The figure shows three views and two pictorial views of one solid part (mm, origin at its lowest corner). Answer the questions. Coordinates: 2 decimals unless noted, no trailing zeros. Write each loop counter-clockwise with the first axis right and the second up, starting at its lowest first coordinate (ties: lowest second). Pieces come first, ordered by that corner, then holes.
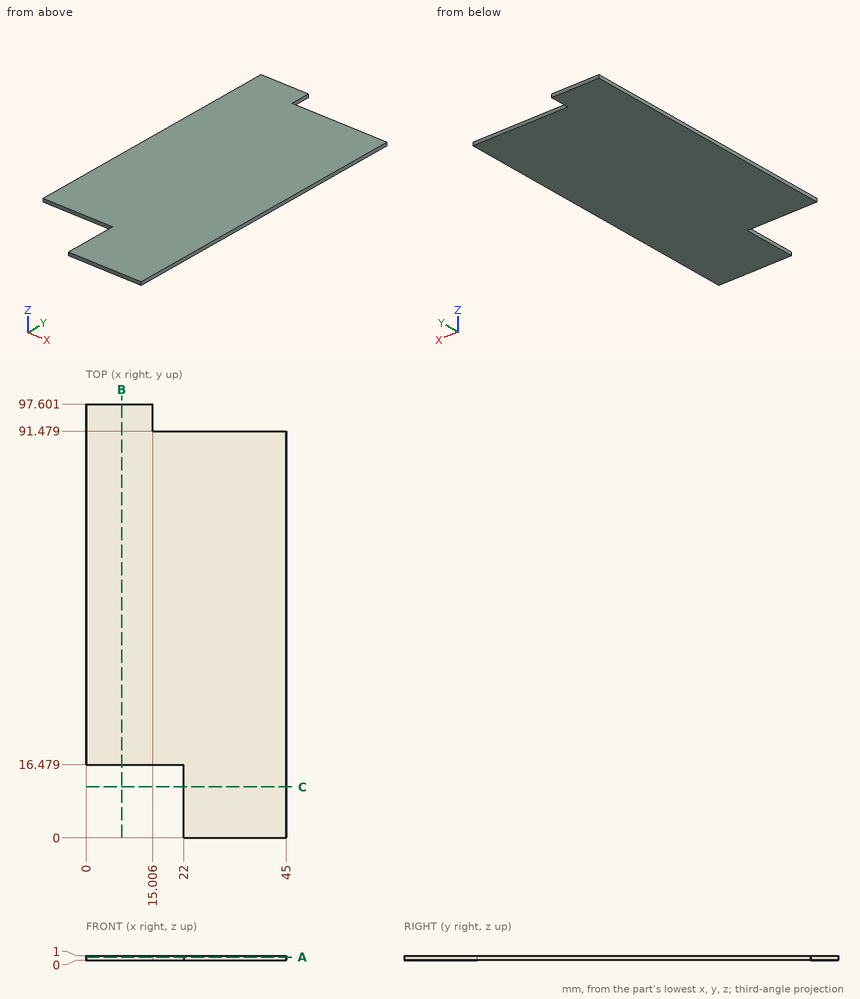
Q1. The part is cut by section A-A, the plane z = 0.75. Write down the section's boundary in (x, y).
Answers below:
outline: (0, 16.48) - (22, 16.48) - (22, 0) - (45, 0) - (45, 91.48) - (15.01, 91.48) - (15.01, 97.6) - (0, 97.6) - close
Q2. Find the intervals of material crossed by probe 1 along Y at (x, z) = (31.5, 0.1); probe 2 along Y at (x, z) = (12, 0.3), in increasing order.
Answers below:
probe 1: y = 0 to 91.48
probe 2: y = 16.48 to 97.6
Q3. The part is cut by section C-C, the plane y = 11.5. Write down the section's boundary in (x, z).
Answers below:
outline: (22, 0) - (45, 0) - (45, 1) - (22, 1) - close
Q4. Given pin 1 (0.5 mm diameter, centred on x = 27, z = 0.5, fed in from +Y); pin 2 (0.5 mm diameter, centred on y = 7.5, z = 0.5, fed in from -X), each flat-ended and moving along its own axis, determine where each tip first touches the part or whether it passes through.
Answers below:
pin 1: stops at y = 91.48
pin 2: stops at x = 22
Q5. The part is cut by section B-B, the plane x = 8. Write down the section's boundary in (y, z).
Answers below:
outline: (16.48, 0) - (97.6, 0) - (97.6, 1) - (16.48, 1) - close
